Design review of the part built by this model. Coordinates are the model's own, in mm. A direction names the side the tool comes from. Give positions to 0.01 mm unless a question says otherwise; leave off trailing zeros. Write each loop counter-clockwise with the first axis right and the second up, starting at its lowest first coordinate (ties: lowest second). Pieces come first, ordered by that corner, then holes. Notation, with made-up numbers: M 30.5,-13.5 L 81.5,-13.5 A31 cw 81.5,15.5 Z; hole C 33,80 d10. An arc over 180 degrees is marked long. Answer in a Markdown table with one row per item.
```python
from build123d import *

# Parameters (mm, degrees)
F0_W       = 10
F0_H       = 3.305
F0_W_2     = 71.45
F0_W_3     = 8.75
F0_H_2     = 10.025
F0_W_4     = 9.8
F1_DEPTH   = 4
F2_DEPTH   = 13.5
F3_DEPTH   = 23.6
F4_SIZE2   = 10
F4_SIZE    = 16
F4_2_SIZE2 = 10
F4_2_SIZE  = 16
F6_DEPTH   = 40.151
F7_R       = 4.25
F8_DEPTH   = 25
F10_DEPTH  = 18.5


with BuildPart() as f1:
    # F0 (on Top) → F1 (new body)
    with BuildSketch(Plane.XY):
        with Locations((32.1862275445, -12.024865455)):
            Rectangle(F0_W, F0_H)
        with Locations((-17.2887724555, -12.024865455)):
            Rectangle(F0_W_2, F0_H)
        with Locations((22.8112275445, -12.024865455)):
            Rectangle(F0_W_3, F0_H)
        with Locations((22.8112275445, -18.689865455)):
            Rectangle(F0_W_3, F0_H_2)
        with Locations((32.1862275445, -18.689865455)):
            Rectangle(F0_W, F0_H_2)
        with Locations((-17.2887724555, -18.689865455)):
            Rectangle(F0_W_2, F0_H_2)
        with Locations((-57.9137724555, -18.689865455)):
            Rectangle(F0_W_4, F0_H_2)
        with Locations((-57.9137724555, -12.024865455)):
            Rectangle(F0_W_4, F0_H)
        with Locations((-57.9137724555, 4.770134545)):
            Rectangle(F0_W_4, F0_H)
        with Locations((-57.9137724555, 11.435134545)):
            Rectangle(F0_W_4, F0_H_2)
        with Locations((-17.2887724555, 11.435134545)):
            Rectangle(F0_W_2, F0_H_2)
        with Locations((-17.2887724555, 4.770134545)):
            Rectangle(F0_W_2, F0_H)
        with Locations((22.8112275445, 11.435134545)):
            Rectangle(F0_W_3, F0_H_2)
        with Locations((22.8112275445, 4.770134545)):
            Rectangle(F0_W_3, F0_H)
        with Locations((32.1862275445, 4.770134545)):
            Rectangle(F0_W, F0_H)
        with Locations((32.1862275445, 11.435134545)):
            Rectangle(F0_W, F0_H_2)
        Polygon((37.1862275445, 3.117634545), (27.1862275445, 3.117634545), (27.1862275445, -3.627365455), (27.1862275445, -10.372365455), (37.1862275445, -10.372365455), align=None)
    extrude(amount=-F1_DEPTH)

    # F0 (on Top) → F2 (join)
    with BuildSketch(Plane.XY):
        with Locations((-57.9137724555, -18.689865455)):
            Rectangle(F0_W_4, F0_H_2)
        with Locations((-17.2887724555, -18.689865455)):
            Rectangle(F0_W_2, F0_H_2)
        with Locations((22.8112275445, -18.689865455)):
            Rectangle(F0_W_3, F0_H_2)
        with Locations((32.1862275445, -18.689865455)):
            Rectangle(F0_W, F0_H_2)
        with Locations((32.1862275445, 11.435134545)):
            Rectangle(F0_W, F0_H_2)
        with Locations((22.8112275445, 11.435134545)):
            Rectangle(F0_W_3, F0_H_2)
        with Locations((-17.2887724555, 11.435134545)):
            Rectangle(F0_W_2, F0_H_2)
        with Locations((-57.9137724555, 11.435134545)):
            Rectangle(F0_W_4, F0_H_2)
    extrude(amount=-F2_DEPTH)

    # F0 (on Top) → F3 (join)
    with BuildSketch(Plane.XY):
        Polygon((-53.0137724555, 3.117634545), (-62.8137724555, 3.117634545), (-62.8137724555, -10.372365455), (-53.0137724555, -10.372365455), (-53.0137724555, -3.627365455), align=None)
        with Locations((-57.9137724555, -12.024865455)):
            Rectangle(F0_W_4, F0_H)
        with Locations((-57.9137724555, -18.689865455)):
            Rectangle(F0_W_4, F0_H_2)
        with Locations((-57.9137724555, 4.770134545)):
            Rectangle(F0_W_4, F0_H)
        with Locations((-57.9137724555, 11.435134545)):
            Rectangle(F0_W_4, F0_H_2)
        with Locations((32.1862275445, 11.435134545)):
            Rectangle(F0_W, F0_H_2)
        with Locations((22.8112275445, 4.770134545)):
            Rectangle(F0_W_3, F0_H)
        with Locations((22.8112275445, 11.435134545)):
            Rectangle(F0_W_3, F0_H_2)
        Polygon((27.1862275445, 3.117634545), (18.4362275445, 3.117634545), (18.4362275445, -3.627365455), (18.4362275445, -10.372365455), (27.1862275445, -10.372365455), (27.1862275445, -3.627365455), align=None)
        with Locations((22.8112275445, -18.689865455)):
            Rectangle(F0_W_3, F0_H_2)
        with Locations((22.8112275445, -12.024865455)):
            Rectangle(F0_W_3, F0_H)
        with Locations((32.1862275445, -18.689865455)):
            Rectangle(F0_W, F0_H_2)
        with Locations((32.1862275445, -12.024865455)):
            Rectangle(F0_W, F0_H)
        Polygon((37.1862275445, 3.117634545), (27.1862275445, 3.117634545), (27.1862275445, -3.627365455), (27.1862275445, -10.372365455), (37.1862275445, -10.372365455), align=None)
        with Locations((32.1862275445, 4.770134545)):
            Rectangle(F0_W, F0_H)
    extrude(amount=F3_DEPTH)

    # F4
    f4_edges = [f1.edges().sort_by_distance(p)[0] for p in [
        (-57.913772, 16.447635, 23.6),
    ]]
    f4_side = f1.faces().sort_by_distance((-9.085188, 16.447635, -0.574122))[0]
    chamfer(f4_edges, length=F4_SIZE, length2=F4_SIZE2, reference=f4_side)

    # F4#2
    f4_2_edges = [f1.edges().sort_by_distance(p)[0] for p in [
        (-57.913772, -23.702365, 23.6),
    ]]
    f4_2_side = f1.faces().sort_by_distance((-9.085188, -23.702365, -0.574122))[0]
    chamfer(f4_2_edges, length=F4_2_SIZE, length2=F4_2_SIZE2, reference=f4_2_side)

    # F5 (on face) → F6 (cut, through all)
    with BuildSketch(Plane(origin=(0, 16.447634545, 0), x_dir=(-1, 0, 0), z_dir=(0, 1, 0))):
        with BuildLine():
            ThreePointArc((-37.1862275445, 0.3616424249), (-34.1889830456, 13.252952829), (-25.9362275445, 23.6))
            Line((-25.9362275445, 23.6), (-37.1862275445, 23.6))
            Line((-37.1862275445, 23.6), (-37.1862275445, 0.3616424249))
        make_face()
    extrude(amount=-F6_DEPTH, mode=Mode.SUBTRACT)

    # F7 (on face) → F8 (cut)
    with BuildSketch(Plane(origin=(-62.8137724555, 0, 0), x_dir=(0, -1, 0), z_dir=(-1, 0, 0))):
        with Locations((3.627365455, 12.6)):
            Circle(F7_R)
    extrude(amount=-F8_DEPTH, mode=Mode.SUBTRACT)

    # F9 (on face) → F10 (cut)
    with BuildSketch(Plane.XY.offset(23.6)):
        Polygon((-54.9137724555, -10.877365455), (-54.9137724555, -3.627365455), (-54.9137724555, 3.622634545), (-57.9137724555, 3.622634545), (-60.9137724555, 3.622634545), (-60.9137724555, -3.627365455), (-60.9137724555, -10.877365455), (-57.9137724555, -10.877365455), align=None)
    extrude(amount=-F10_DEPTH, mode=Mode.SUBTRACT)


solid = f1.part
```
1) Add section D-D (z = -1.5). Write out the cut boundary in (x, y).
Geometry says:
| item | result |
|---|---|
| outline | M -62.81,-23.7 L 37.19,-23.7 L 37.19,16.45 L -62.81,16.45 L -62.81,3.12 L 27.19,3.12 L 27.19,-10.37 L -62.81,-10.37 Z |
2) To check wall thickness, follow probe 1 along Y at (x, z) = (-12, -2); probe 2 along X at (y, z) = (-9, 9.5); probe 3 along X at (y, z) = (-9, 7.5). State the ranges of each line that lie inside material, in increasing order. Write a range as [from, to].
Geometry says:
| item | result |
|---|---|
| probe 1 | [-23.7, -10.37], [3.12, 16.45] |
| probe 2 | [-62.81, -60.91], [-54.91, -53.01], [18.44, 35.7] |
| probe 3 | [-62.81, -60.91], [-54.91, -53.01], [18.44, 36.28] |
3) The part is to be moulded in two halves that separate along Z. For faces 1 (the face through (-61.88, -2.71, 8.45)), 2 (the face through (-2, 5, -4)), 3 (the face through (-2, 16.448, -3)), say which applies: released by +Z, released by -Z, zero draft, split by the parting line, or undercut.
Geometry says:
| item | result |
|---|---|
| face 1 | undercut |
| face 2 | released by -Z |
| face 3 | zero draft |
4) For faces 4 (the face through (-60.914, -2, 17)), 5 (the face through (18.436, -3, 12)), 6 (the face through (-53.98, -2.71, 8.45)), list the 3-axis set-ups (+Z, -Z, +X, -X, +Y, -Y) from which the entire face can be reached by the end or side of a thin tool; tool diameter is ignored.
Geometry says:
| item | result |
|---|---|
| face 4 | +Z |
| face 5 | +Z, +Y, -Y |
| face 6 | -X |
5) Insertion check: P1, Ø11, axis at x = -58.5, y = -4.5, coming from the -Z side; P2, Ø12, axis at y = 2, z = 7, coming from the +X side; P3, Ø4.5, axis at y = -1, z = 15, coming from the +X side. Each pin has a flat end and moves straight along its axis. Give the tip position at first contact, or say it passes through.
Geometry says:
| item | result |
|---|---|
| P1 | z = 0 |
| P2 | x = 37.18 |
| P3 | x = 34.43 |
6) Add section C-C (z = -9.5). Write out the cut boundary in (x, y), and give its area (4 significant figures).
Geometry says:
| item | result |
|---|---|
| outline | M -62.81,-23.7 L 37.19,-23.7 L 37.19,-13.68 L -62.81,-13.68 Z; M -62.81,6.42 L 37.19,6.42 L 37.19,16.45 L -62.81,16.45 Z |
| area | 2,005 mm^2 |
7) Add section B-B (x = -38). Write out the cut boundary in (y, z).
Geometry says:
| item | result |
|---|---|
| outline | M -23.7,-13.5 L -13.68,-13.5 L -13.68,-4 L -10.37,-4 L -10.37,0 L -23.7,0 Z; M 3.12,-4 L 6.42,-4 L 6.42,-13.5 L 16.45,-13.5 L 16.45,0 L 3.12,0 Z |
8) Add section A-A (z = 19.5). Write out the cut boundary in (x, y).
Geometry says:
| item | result |
|---|---|
| outline | M -62.81,-16.26 L -53.01,-16.26 L -53.01,9.01 L -62.81,9.01 Z; M 18.44,-23.7 L 30.14,-23.7 L 30.14,16.45 L 18.44,16.45 Z; hole M -60.91,-10.88 L -54.91,-10.88 L -54.91,3.62 L -60.91,3.62 Z |
